Part print with two shaded views. Sizes in mm from the minimum x, y, z corner. A direction names the side the tool comes from. Coordinates: 2 decimals unless noted, no trailing zeros. Order: outer loops, then holes, each group sorted by start corner. A loop starts at its lowest first (then second) coordinate and runs counter-clockwise, first axis right, second up. Notation, with made-up numbers: (-28.5, 7) - (-16.5, 7) arc R25 ccw to (-16.5, 21) - close; hole circle Ø3 at (-36.5, 79.25). An arc over 180 degrees is marked (long way). One line per item, written item: value.
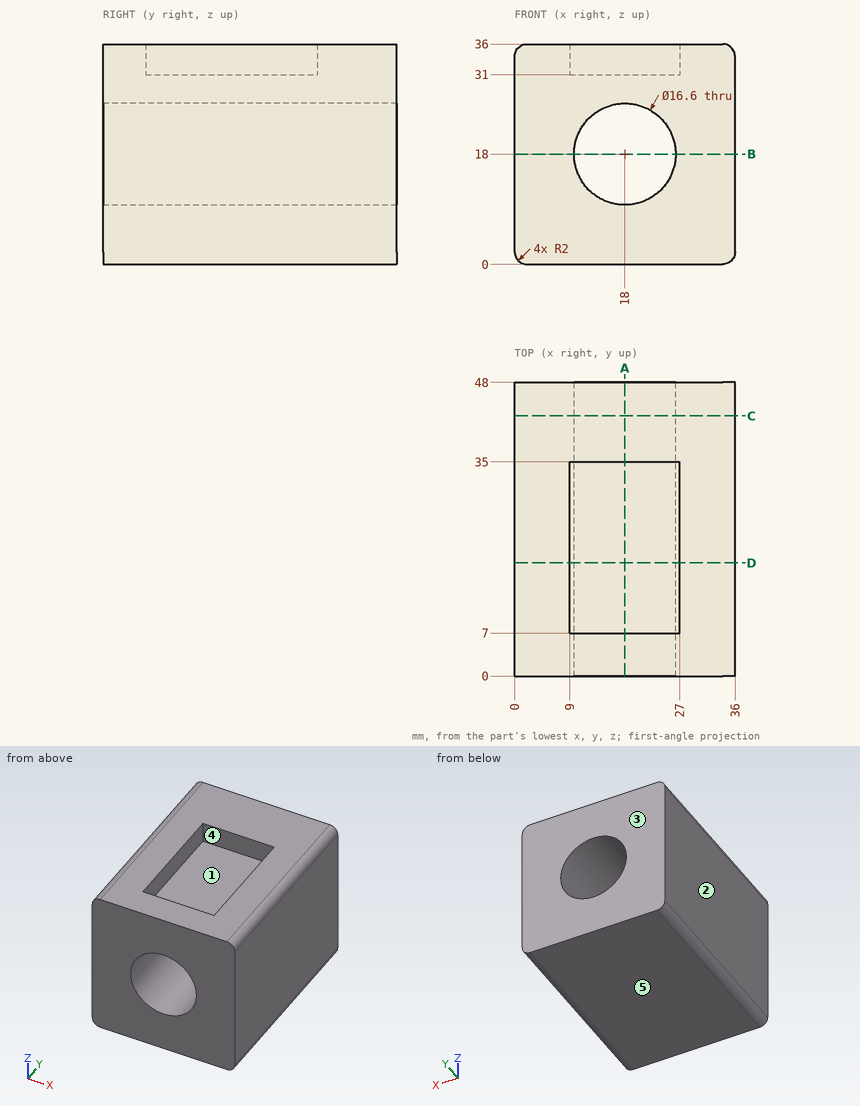
1. Band-saw the part on B-B, the plane z = 18. Give the cut face in (x, y).
Values found:
outline: (0, 0) - (9.7, 0) - (9.7, 48) - (0, 48) - close; (26.3, 0) - (36, 0) - (36, 48) - (26.3, 48) - close
2. Probe line 1 along Y through (x, z) = (11.5, 32); line 2 along X through (y, z) = (23, 18); line 3 along Z through (x, y) = (24.5, 41). List the from-to ranges inside material, lowest first.
Values found:
line 1: y = 0 to 7, 35 to 48
line 2: x = 0 to 9.7, 26.3 to 36
line 3: z = 0 to 12.84, 23.16 to 36
3. 3-axis set-ups, long thin cutter, end or side, ignore diameter. For the marked faces 4 and 5: which of +Z, -Z, +X, -X, +Y, -Y reach the whole face in a straight line?
Values found:
face 4: +Z
face 5: -Z, +X, -X, +Y, -Y
4. Flat gauge pins, fed straight in: P1, Ø3, axis at x = 14, z = 13.5, coming from the -Y side; P2, Ø5.5, axis at x = 19.5, y = 20, coming from the +Z side. Where does each tip first touch, or does it go through?
Values found:
P1: passes through
P2: stops at z = 31
5. Band-saw the part on D-D, the plane y = 18.5. Give the cut face in (x, z).
Values found:
outline: (0, 2) arc R2 ccw to (2, 0) - (34, 0) arc R2 ccw to (36, 2) - (36, 34) arc R2 ccw to (34, 36) - (27, 36) - (27, 31) - (9, 31) - (9, 36) - (2, 36) arc R2 ccw to (0, 34) - close; hole circle Ø16.6 at (18, 18)
6. Two-plate mould, pull along Y, no slides. Class the marked faces 1, 2 and 3: pulls with the +Y half, pulls with the -Y half, needs draft (parallel to the pull), parting line crosses it, or undercut.
Values found:
face 1: undercut
face 2: needs draft
face 3: pulls with the +Y half
7. Band-saw the part on A-A, the plane x = 18. Give the cut face in (y, z).
Values found:
outline: (0, 0) - (48, 0) - (48, 9.7) - (0, 9.7) - close; (0, 26.3) - (48, 26.3) - (48, 36) - (35, 36) - (35, 31) - (7, 31) - (7, 36) - (0, 36) - close
8. Band-saw the part on C-C, the plane y = 42.5. Give the cut face in (x, z).
Values found:
outline: (0, 2) arc R2 ccw to (2, 0) - (34, 0) arc R2 ccw to (36, 2) - (36, 34) arc R2 ccw to (34, 36) - (2, 36) arc R2 ccw to (0, 34) - close; hole circle Ø16.6 at (18, 18)
